Check sheet for the drawn part. Datum: minimum x, y, z corner. Units: mm. Round coordinates to 2 decimals unless told otherwise and drop trailing zeros. Write each loop counter-clockwise with the first axis right and the second up, starting at its lowest first coordinate (ties: lowest second). Pieces come first, ordered by that corner, then holes. Notation, with made-up numbers: (4.25, -24) - (59.25, -24) arc R32 ccw to (59.25, 12) - close; hole circle Ø4 at (12, -2). An arc over 180 degrees is marked (long way). Write each question's results on one line, items separated by ' | '.
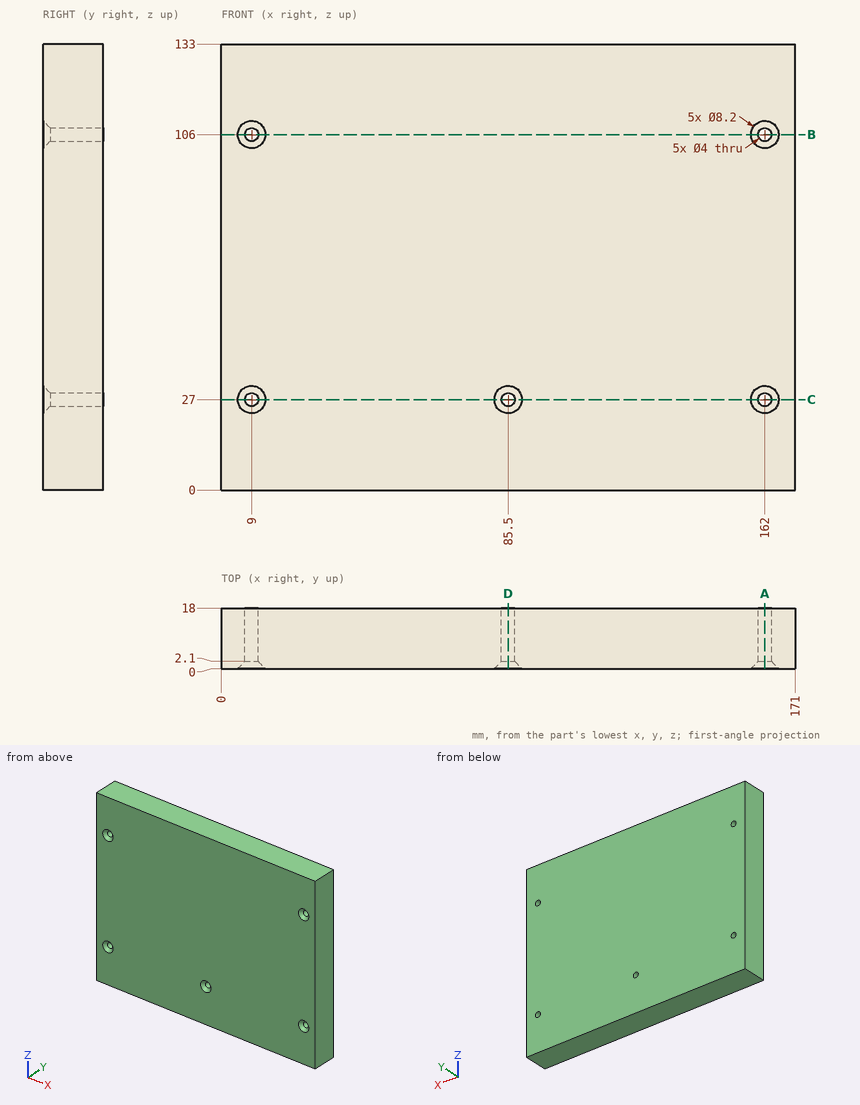
(1) Section check C-C (z = 27). Record the cut outline in (x, y), plus the area to 3 significant figures.
Answer:
outline: (0, 0) - (4.9, 0) - (7, 2.1) - (7, 18) - (0, 18) - close; (11, 2.1) - (13.1, 0) - (81.4, 0) - (83.5, 2.1) - (83.5, 18) - (11, 18) - close; (87.5, 2.1) - (89.6, 0) - (157.9, 0) - (160, 2.1) - (160, 18) - (87.5, 18) - close; (164, 2.1) - (166.1, 0) - (171, 0) - (171, 18) - (164, 18) - close | area: 2,850 mm2
(2) Section check B-B (z = 106). Record the cut outline in (x, y).
Answer:
outline: (0, 0) - (4.9, 0) - (7, 2.1) - (7, 18) - (0, 18) - close; (11, 2.1) - (13.1, 0) - (157.9, 0) - (160, 2.1) - (160, 18) - (11, 18) - close; (164, 2.1) - (166.1, 0) - (171, 0) - (171, 18) - (164, 18) - close
(3) Thickness scan on L1, parallel to X at y = 12.25, z = 27; L2, parallel to Z at x = 162, y = 12; L3, parallel to X at y = 8.25, z = 106. Record the ranges inside material, lowest first.
Answer:
L1: 0 to 7, 11 to 83.5, 87.5 to 160, 164 to 171 | L2: 0 to 25, 29 to 104, 108 to 133 | L3: 0 to 7, 11 to 160, 164 to 171
(4) Section check D-D (x = 85.5). Record the cut outline in (y, z).
Answer:
outline: (0, 0) - (18, 0) - (18, 25) - (2.1, 25) - (0, 22.9) - close; (0, 31.1) - (2.1, 29) - (18, 29) - (18, 133) - (0, 133) - close
(5) Go/stop test with flat-tipped pins: pin 1 Ø3.5 at (x, z) = (85.5, 27) entering from -Y; pin 2 Ø3 at (x, z) = (40.5, 85.5) entering from -Y. Record where each tip stops, or that it passes through.
Answer:
pin 1: through | pin 2: y = 0
(6) Section check A-A (x = 162). Record the cut outline in (y, z).
Answer:
outline: (0, 0) - (18, 0) - (18, 25) - (2.1, 25) - (0, 22.9) - close; (0, 31.1) - (2.1, 29) - (18, 29) - (18, 104) - (2.1, 104) - (0, 101.9) - close; (0, 110.1) - (2.1, 108) - (18, 108) - (18, 133) - (0, 133) - close
